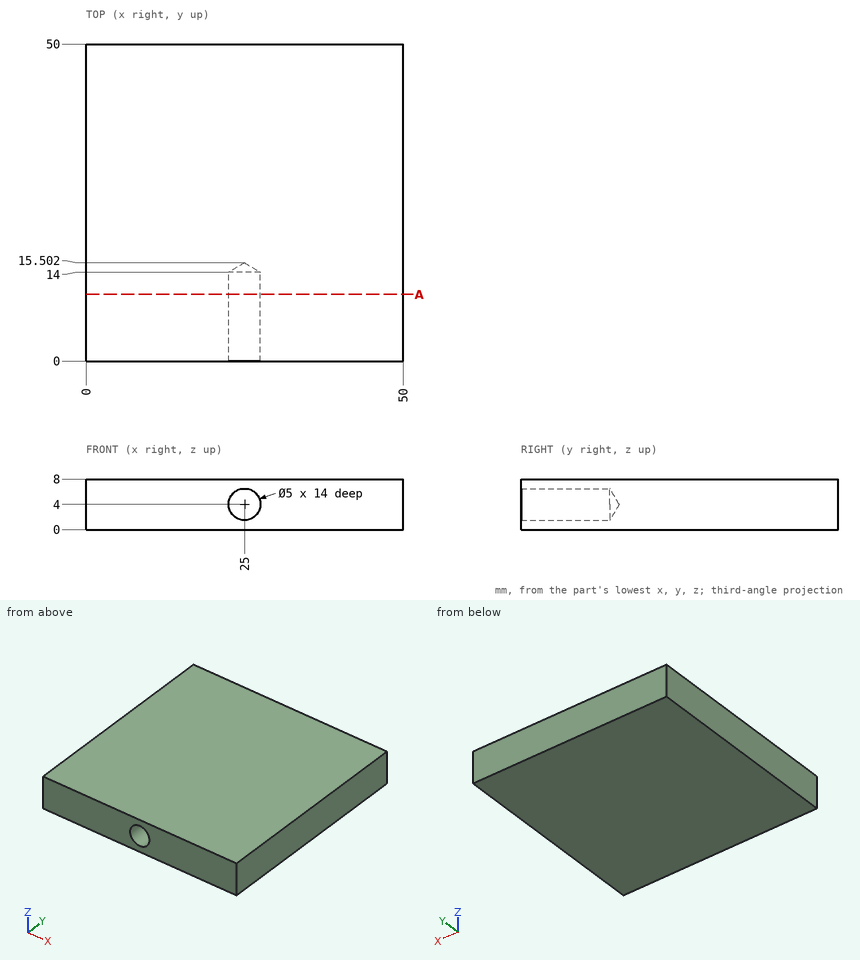
Input: dimensioned drawing with shaded views. Units: mm. Origin: part minimum x, y, z. Round coordinates to 2 decimals unless told otherwise and drop trailing zeros. Loops run counter-clockwise (first coordinate to the right, second up) from the corner with the lowest first, then second, coordinate; pieces in that order, holes last. Notation, with made-up numbers: (17, 70.25) -> (46, 70.25) arc R24 cw to (46, 101.25) -> close; hole circle Ø9 at (85, 53). An arc over 180 degrees is marked (long way). Answer as a JSON object with one key per item and string values. Group by question number.
Q1. Ray query, line 1 (Z direction, x = 25, y = 5.75); line 2 (X direction, y = 10, z = 5); line 3 (X direction, y = 14, z = 3.5). Return the intervals inside material, ascending. Write a range as from..to.
Q2. Contact query for a flat-ended pin moving along its axis: P1, Ø3, axis at x = 25, z = 4, coming from the -Y side. Output: stop coordinate, or through.
Q3. Section query A-A (y = 10.5). Output: boundary loops of the cut face in (x, z), plus the area to 3 significant figures.
Completed:
{
 "1": {"line 1": "0..1.5, 6.5..8", "line 2": "0..22.71, 27.29..50", "line 3": "0..22.55, 27.45..50"},
 "2": {"P1": "y = 14.6"},
 "3": {"outline": "(0, 0) -> (50, 0) -> (50, 8) -> (0, 8) -> close; hole circle Ø5 at (25, 4)", "area": "380 mm²"}
}
